```python
from build123d import *

# Parameters (mm, degrees)
BOSS_EXTRUDE2_REACH             = 37.299
BOSS_EXTRUDE2_END_RADIUS        = 15
BOSS_EXTRUDE2_DIRECTION_2_DEPTH = 40
SKETCH3_R                       = 3.25
CUT_EXTRUDE1_DEPTH              = 35
SKETCH4_R                       = 1.25
CUT_EXTRUDE3_DEPTH              = 2
CUT_EXTRUDE4_REACH              = 62.092
CUT_EXTRUDE4_END_RADIUS         = 3.25
SKETCH4_3_R                     = 1.25


with BuildPart() as part:
    # Sketch1 → Revolve1 (revolve)
    with BuildSketch(Plane.XY):
        with BuildLine():
            Line((9.604686356, 8), (12.68857754, 8))
            ThreePointArc((12.68857754, 8), (14.872770572, -1.949537258), (10.198039027, -11))
            Line((10.198039027, -11), (5.937171044, -11))
            ThreePointArc((5.937171044, -11), (12.27344014, -2.369106824), (9.604686356, 8))
        make_face()
    revolve(axis=Axis((0, 10, 0), (0, -1, 0)))

    # Boss-Extrude2: up to this sphere (the profile starts outside it)
    boss_extrude2_end = Location((0, 0, 0)) * Sphere(BOSS_EXTRUDE2_END_RADIUS, mode=Mode.PRIVATE)
    # Sketch2 → Boss-Extrude2 (add, up to the surface)
    with BuildSketch(Plane(origin=(0, 0, -15), x_dir=(-1, 0, 0), z_dir=(0, 0, -1)), mode=Mode.PRIVATE) as boss_extrude2_sk1:
        with BuildLine():
            Line((4.123105626, 8), (-4.123105626, 8))
            ThreePointArc((-4.123105626, 8), (0, -9), (4.123105626, 8))
        make_face()
    boss_extrude2_tool1 = extrude(boss_extrude2_sk1.sketch, amount=-BOSS_EXTRUDE2_REACH, mode=Mode.PRIVATE) - boss_extrude2_end
    add(boss_extrude2_tool1.solids().sort_by_distance((0, -0.187735, -15))[0])

    # Sketch2 → Boss-Extrude2 direction 2 (add)
    with BuildSketch(Plane(origin=(0, 0, -15), x_dir=(-1, 0, 0), z_dir=(0, 0, -1))):
        with BuildLine():
            Line((4.123105626, 8), (-4.123105626, 8))
            ThreePointArc((-4.123105626, 8), (0, -9), (4.123105626, 8))
        make_face()
    extrude(amount=BOSS_EXTRUDE2_DIRECTION_2_DEPTH)

    # Sketch3 → Cut-Extrude1 (cut)
    with BuildSketch(Plane(origin=(0, 0, -55), x_dir=(-1, 0, 0), z_dir=(0, 0, -1))):
        Circle(SKETCH3_R)
    extrude(amount=-CUT_EXTRUDE1_DEPTH, mode=Mode.SUBTRACT)

    # Sketch4 → Cut-Extrude3 (cut)
    # profile 1 of 2: a face of its own
    with BuildSketch(Plane(origin=(0, 8, 0), x_dir=(1, 0, 0), z_dir=(0, 1, 0))):
        Polygon((-2, 26.845299462), (0, 25.690598923), (2, 26.845299462), (2, 29.154700538), (0, 30.309401077), (-2, 29.154700538), align=None)
        with Locations(Location((0, 28, 0), (0, 0, 180))):
            Circle(SKETCH4_R, mode=Mode.SUBTRACT)
    # profile 2 of 2: a face of its own
    with BuildSketch(Plane(origin=(0, 8, 0), x_dir=(1, 0, 0), z_dir=(0, 1, 0))):
        Polygon((-2, 41.845299462), (0, 40.690598923), (2, 41.845299462), (2, 44.154700538), (0, 45.309401077), (-2, 44.154700538), align=None)
        with Locations(Location((0, 43, 0), (0, 0, 180))):
            Circle(SKETCH4_R, mode=Mode.SUBTRACT)
    extrude(amount=-CUT_EXTRUDE3_DEPTH, mode=Mode.SUBTRACT)

    # Cut-Extrude4: up to this cylinder (the profile starts outside it)
    cut_extrude4_end = Plane(origin=(0, 0, -35.5), z_dir=(0, 0, -1)) * Cylinder(CUT_EXTRUDE4_END_RADIUS, 146.684, mode=Mode.PRIVATE)
    # Sketch4<3> → Cut-Extrude4 (cut, up to the surface)
    with BuildSketch(Plane(origin=(0, 8, 0), x_dir=(1, 0, 0), z_dir=(0, 1, 0)), mode=Mode.PRIVATE) as cut_extrude4_sk1:
        with Locations(Location((0, 28, 0), (0, 0, 180))):
            Circle(SKETCH4_3_R)
    cut_extrude4_tool1 = extrude(cut_extrude4_sk1.sketch, amount=-CUT_EXTRUDE4_REACH, mode=Mode.PRIVATE) - cut_extrude4_end
    add(cut_extrude4_tool1.solids().sort_by_distance((0, 8, -28))[0], mode=Mode.SUBTRACT)
    # Sketch4<3> → Cut-Extrude4 (cut, up to the surface)
    with BuildSketch(Plane(origin=(0, 8, 0), x_dir=(1, 0, 0), z_dir=(0, 1, 0)), mode=Mode.PRIVATE) as cut_extrude4_sk2:
        with Locations(Location((0, 43, 0), (0, 0, 180))):
            Circle(SKETCH4_3_R)
    cut_extrude4_tool2 = extrude(cut_extrude4_sk2.sketch, amount=-CUT_EXTRUDE4_REACH, mode=Mode.PRIVATE) - cut_extrude4_end
    add(cut_extrude4_tool2.solids().sort_by_distance((0, 8, -43))[0], mode=Mode.SUBTRACT)


solid = part.part
```
Check sheet for the modelled part. Datum: model origin and axes. Units: mm. A direction names the side the tool comes from. Round coordinates to 2 decimals unless told otherwise and drop trailing zeros. Write each loop counter-clockwise with the first axis right and the second up, starting at its lowest first coordinate (ties: lowest second). Pieces come first, ordered by that corner, then holes. Notation, with made-up numbers: (-7, 39) -> (50, 39) arc R20 ccw to (50, 62) -> close; hole circle Ø8 at (34, 65). An arc over 180 degrees is marked (long way). Put each result on its own line as item: value.
(1) Mould release check, pull along X, two halves, no side actions. Record for faces 1 (the face through (0, -9, -33)), 2 (the face through (0, -11, -7)), 3 (the face through (-0.99, 7.01, -44.74)): released by +X, released by -X, zero draft, split by the parting line, or undercut.
Values found:
face 1: split by the parting line
face 2: zero draft
face 3: undercut
(2) Sectioned sample at C-C (z = -28). Enter the section's corners in (x, y), plus the area to 3 significant figures.
Values found:
outline: (-4.12, 8) arc R9 ccw (long way) to (4.12, 8) -> (2, 8) -> (2, 6) -> (1.25, 6) -> (1.25, 3) arc R3.25 cw (long way) to (-1.25, 3) -> (-1.25, 6) -> (-2, 6) -> (-2, 8) -> close
area: 201 mm^2
(3) Sectioned sample at B-B (x = 5.25). Enter the section's corners in (y, z).
Values found:
outline: (-11, -8.74) arc R14.05 ccw to (-7.31, -12) -> (-7.31, -55) -> (7.31, -55) -> (7.31, -12) arc R14.05 ccw to (8, -11.55) -> (8, -8.04) arc R11.34 cw to (-11, -2.77) -> close; (-11, 2.77) arc R11.34 cw to (8, 8.04) -> (8, 11.55) arc R14.05 ccw to (-11, 8.74) -> close
(4) Sectioned sample at D-D (z = -36.5). Enter the section's corners in (x, y).
Values found:
outline: (-4.12, 8) arc R9 ccw (long way) to (4.12, 8) -> close; hole circle Ø6.5 at (0, 0)
(5) Tool access check on faces 4 (the face through (2.579, -1.978, -37.745)), 5 (the face through (1.014, 7.014, -44.724)), 6 (the face through (1, 8, -21)). Record the directions out of +Z, -Z, +X, -X, +Y, -Y that give a thin tool (end or side, any length) a straight path to the whole face; none if there is none.
Values found:
face 4: -Z
face 5: +Y
face 6: +Z, -Z, +X, -X, +Y
(6) Sectioned sample at A-A (y = 0). Enter the section's corners in (x, z).
Values found:
outline: (-9, -55) -> (-3.25, -55) -> (-3.25, -20) -> (3.25, -20) -> (3.25, -55) -> (9, -55) -> (9, -12) arc R15 ccw (long way) to (-9, -12) -> close; hole circle Ø25 at (0, 0)
(7) Material ranges on line 1 (X direction, y = 0.25, z = -43); line 2 (Z direction, x = 0, y = 4.5); line 3 (Z direction, x = 0, y = 4.7), recorded low to high.
Values found:
line 1: x = -9 to -3.24, 3.24 to 9
line 2: z = -55 to -44.25, -41.75 to -29.25, -26.75 to -11.66, 11.66 to 14.31
line 3: z = -55 to -44.25, -41.75 to -29.25, -26.75 to -11.58, 11.58 to 14.24
(8) Go/stop test with flat-tipped pins: pin 1 Ø8 at (y, z) = (-6, 6) entering from -X; pin 2 Ø1 at (y, z) = (7, -43) entering from +X; pin 3 Ø8 at (y, z) = (2.5, -11) entering from -X; pin 4 Ø3 at (x, z) = (1, -42) entering from +Y. Record where each tip stops, or that it passes through.
Values found:
pin 1: stops at x = -14.31
pin 2: stops at x = 6.22
pin 3: stops at x = -13.11
pin 4: stops at y = 8
